Source: CAD feature listing. Evaluate the final solid. Frame: model axes, mm. A direction names the side the tool comes from. Give positions to 0.01 mm unless a question says otherwise; leave off trailing zeros. Order: outer loops, then holes, each group sorted by start corner. A loop starts at its lowest first (then second) coordinate and runs counter-clockwise, first axis right, second up. Notation, with made-up numbers: M 37,43 L 78,43 A8 cw 78,58 Z; hole C 63.25,72.25 d5. An arc over 180 degrees is marked long. Answer in a Markdown table with one row per item. Add a question column.
(1) Section query B-B, the plane z = 7.5. Return loops of the section in (x, y), plus the area to 3 significant figures.
(2) Section query A-A, the plane x = 0. Return loops of the section in (y, z).
(3) Mould query, pull axis X, two halves, no side actions, for faces 4 (the face through (0, 1, 8)), 5 (the face through (-1.08, -4.88, 1.24)), 6 (the face through (0.04, -1.61, 2.71)), 7 (the face through (0, -1, 2)). Classes: pulls with the +X half, pulls with the -X half, needs draft (parallel to the pull), parting line crosses it, or undercut.
(4) Section query C-C, the plane z = 2.25. Return loops of the section in (x, y), plus the area to 3 significant figures.
(5) Pin query (flat end, axial travel): P1, Ø1.5, axis at y = -1, z = 1.5, coming from the +X side; P2, Ø4, axis at x = 2, y = -4, coming from the -Z side; P3, Ø1, axis at y = -2, z = 1, coming from the -X side; P4, Ø1.5, axis at x = -0.5, y = -2.5, coming from the +Z side. Return the tip coordinate at first contact, or that it passes through.
(6) Set-up query: faces 1 (the face through (-0.54, -2.44, 2.3)), 2 (the face through (0, 0, 0)), 3 (the face through (0, 1.5, 5.3)). Return all of +Z, -Z, +X, -X, +Y, -Y with unobstructed straight access to the full face (end or side cutting, diameter ignored); none if empty.
(7) Material intervals for line 1 along Z through (x, y) = (-3.75, 0.5); line 2 along Z through (x, y) = (-0.75, 1.75); line 3 along Y through (x, z) = (0, 3.25), sorted ascending.
from build123d import *

# Parameters (mm, degrees)
F2_DEPTH = 8
F1_R     = 2.5
F4_DEPTH = 3
F1_R_2   = 5
F6_DEPTH = 2
F7_DEPTH = 2
F8_SIZE  = 0.4
F9_SIZE  = 0.3
F10_SIZE = 0.5
F11_SIZE = 0.4


with BuildPart() as f2:
    # F1 (on Top) → F2 (new body)
    with BuildSketch(Plane.XY):
        with BuildLine():
            Line((-1.5, 0), (1.5, 0))
            ThreePointArc((1.5, 0), (0, 1.5), (-1.5, 0))
        make_face()
    extrude(amount=F2_DEPTH)

    # F1 (on Top) → F4 (join)
    with BuildSketch(Plane.XY):
        Circle(F1_R)
        with BuildLine():
            ThreePointArc((-1.5, 0), (0, 1.5), (1.5, 0))
            ThreePointArc((1.5, 0), (0, -1.5), (-1.5, 0))
        make_face(mode=Mode.SUBTRACT)
    extrude(amount=F4_DEPTH)

    # F1 (on Top) → F6 (join)
    with BuildSketch(Plane.XY):
        Circle(F1_R_2)
        Circle(F1_R, mode=Mode.SUBTRACT)
    extrude(amount=F6_DEPTH)

    # F1 (on Top) → F7 (join)
    with BuildSketch(Plane.XY):
        with BuildLine():
            ThreePointArc((-1.5, 0), (0, -1.5), (1.5, 0))
            Line((1.5, 0), (-1.5, 0))
        make_face()
    extrude(amount=F7_DEPTH)

    # F8
    f8_edges = [f2.edges().sort_by_distance(p)[0] for p in [
        (-2.5, 0, 3),
    ]]
    chamfer(f8_edges, length=F8_SIZE)

    # F9
    f9_edges = [f2.edges().sort_by_distance(p)[0] for p in [
        (0, 1.5, 8),
        (0, 0, 8),
    ]]
    chamfer(f9_edges, length=F9_SIZE)

    # F10
    f10_edges = [f2.edges().sort_by_distance(p)[0] for p in [
        (-5, 0, 0),
    ]]
    chamfer(f10_edges, length=F10_SIZE)

    # F11
    f11_edges = [f2.edges().sort_by_distance(p)[0] for p in [
        (0, -1.5, 3),
    ]]
    chamfer(f11_edges, length=F11_SIZE)


solid = f2.part
Values follow:
| question | item | result |
|---|---|---|
| 1 | outline | M -1.5,0 L 1.5,0 A1.5 ccw Z |
| 1 | area | 3.53 mm² |
| 2 | outline | M -5,0.5 L -4.5,0 L 4.5,0 L 5,0.5 L 5,2 L 2.5,2 L 2.5,2.6 L 2.1,3 L 1.5,3 L 1.5,7.7 L 1.2,8 L 0.3,8 L 0,7.7 L 0,2 L -1.5,2 L -1.5,2.6 L -1.9,3 L -2.1,3 L -2.5,2.6 L -2.5,2 L -5,2 Z |
| 3 | face 4 | needs draft |
| 3 | face 5 | parting line crosses it |
| 3 | face 6 | undercut |
| 3 | face 7 | undercut |
| 4 | outline | C 0,0 d5; hole M -1.5,0 A1.5 ccw 1.5,0 Z |
| 4 | area | 16.1 mm² |
| 5 | P1 | stops at x = 4.99 |
| 5 | P2 | stops at z = 0 |
| 5 | P3 | stops at x = -4.77 |
| 5 | P4 | stops at z = 3 |
| 6 | face 1 | +Z |
| 6 | face 2 | -Z, +X, -X, +Y, -Y |
| 6 | face 3 | +Z, +Y |
| 7 | line 1 | z = 0 to 2 |
| 7 | line 2 | z = 0 to 3 |
| 7 | line 3 | y = 0 to 1.5 |
